from build123d import *

# Parameters (mm, degrees)
SKETCH2_R           = 6
BOSS_EXTRUDE1_DEPTH = 10
SKETCH3_W           = 75
SKETCH3_H           = 10
BOSS_EXTRUDE2_DEPTH = 60
SKETCH4_R           = 2.25
CUT_EXTRUDE1_DEPTH  = 9
SKETCH5_W           = 10
SKETCH5_H           = 10
CUT_EXTRUDE2_DEPTH  = 2.5


with BuildPart() as part:
    # Sketch2 → Boss-Extrude1 (new body)
    with BuildSketch(Plane.XY):
        with BuildLine():
            Line((-37.5, -5), (37.5, -5))
            Line((37.5, -5), (37.5, 5))
            Line((37.5, 5), (5.548671219, 35.763006828))
            ThreePointArc((5.548671219, 35.763006828), (0, 38), (-5.548671219, 35.763006828))
            Line((-5.548671219, 35.763006828), (-37.5, 5))
            Line((-37.5, 5), (-37.5, -5))
        make_face()
        with Locations((0, 30)):
            Circle(SKETCH2_R, mode=Mode.SUBTRACT)
    extrude(amount=BOSS_EXTRUDE1_DEPTH)

    # Sketch3 → Boss-Extrude2 (add)
    with BuildSketch(Plane.XY):
        Rectangle(SKETCH3_W, SKETCH3_H)
    extrude(amount=BOSS_EXTRUDE2_DEPTH)

    # Sketch4 → Cut-Extrude1 (cut)
    with BuildSketch(Plane.XZ.offset(5)):
        with Locations((27.5, 5)):
            Circle(SKETCH4_R)
        with Locations((12.5, 5)):
            Circle(SKETCH4_R)
        with Locations((-12.5, 5)):
            Circle(SKETCH4_R)
        with Locations((-27.5, 5)):
            Circle(SKETCH4_R)
    extrude(amount=-CUT_EXTRUDE1_DEPTH, mode=Mode.SUBTRACT)

    # Sketch5 → Cut-Extrude2 (cut)
    with BuildSketch(Plane(origin=(0, 0, 0), x_dir=(-1, 0, 0), z_dir=(0, 0, -1))):
        with Locations((-10, 5)):
            Rectangle(SKETCH5_W, SKETCH5_H)
        with Locations((10, 5)):
            Rectangle(SKETCH5_W, SKETCH5_H)
    extrude(amount=-CUT_EXTRUDE2_DEPTH, mode=Mode.SUBTRACT)


solid = part.part
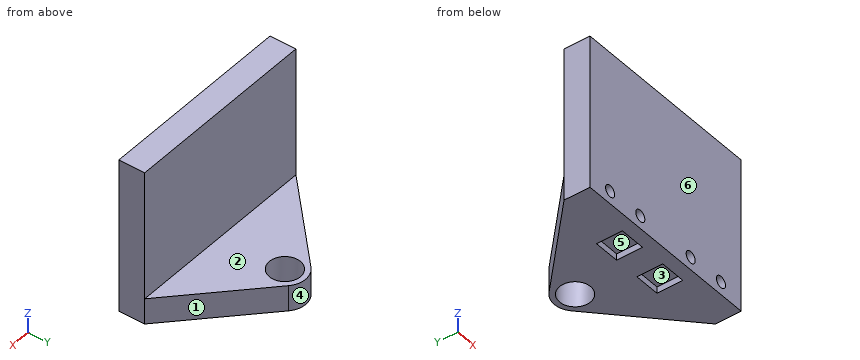
Here's how the part is built. I have some questions about the finished solid (model axes, mm). Face numbers are marked on the shaded views. A direction names the side the tool comes from. Give positions to 0.01 mm unless a question says otherwise; leave off trailing zeros. Loops run counter-clockwise (first coordinate to the right, second up) from the corner with the lowest first, then second, coordinate; pieces in that order, holes last. Notation, with made-up numbers: (57.25, -30.75) -> (85.25, -30.75) arc R31 ccw to (85.25, 7.25) -> close; hole circle Ø10 at (72, 40). An arc over 180 degrees is marked (long way). Answer as a JSON object with one key per item and string values. Group by question number.
Item 1: On a 3-axis mill with a long thin cutter (end or side, diameter ignored), from which of +Z, -Z, +X, -X, +Y, -Y can I reach the whole of each face in a straight line? I mean the marked faces 1, 2 and 3. Say none if no direction works.
Item 2: Imagine slicing it at D-D on x = 27.5. Write out the boundary of the cut face in (y, z).
Item 3: Thinking about a two-plate mould opening in X: for the marked faces 4, 5 and 6, which applies, pulls with the +X half, pulls with the -X half, needs draft (parallel to the pull), parting line crosses it, or undercut?
Item 4: Imagine slicing it at B-B on z = 5. Write out the boundary of the cut face in (x, y), then the cut area to 3 significant figures.
Item 5: Imagine slicing it at C-C on y = 27. Write out the boundary of the cut face in (x, z).
Item 6: Imagine slicing it at A-A on x = 0. Write out the boundary of the cut face in (y, z), then the cut area to 3 significant figures.
Item 7: Will these pins go through, and if not, where does the flat tip stop? pin 1 (2.5 mm diameter, centred on x = 27.5, z = 5, fed in from -Y); pin 2 (4 mm diameter, centred on x = -27.5, z = 5, fed in from +Y); pin 3 (1.5 mm diameter, centred on x = 12.5, y = 25.5, fed in from +Z); pin 4 (9.5 mm diameter, centred on x = 0, y = 30, fed in from -Z).
Item 8: I need wall thicknesses on L1, parallel to Z at x = -12.5, y = -0.75; L2, parallel to Z at x = -12.5, y = 1; L3, parallel to Y at x = -9.5, z = 53.5. Which ranges of each line are inside material? Lowest first, please.
Answer list:
{
 "1": {"face 1": "+Z, -Z, +X, +Y", "face 2": "+Z, +X, -X, +Y", "face 3": "-Z"},
 "2": {"outline": "(-5, 0) -> (14.63, 0) -> (14.63, 10) -> (5, 10) -> (5, 60) -> (-5, 60) -> (-5, 7.25) -> (4, 7.25) -> (4, 2.75) -> (-5, 2.75) -> close"},
 "3": {"face 4": "parting line crosses it", "face 5": "undercut", "face 6": "needs draft"},
 "4": {"outline": "(-37.5, -5) -> (-29.75, -5) -> (-29.75, 4) -> (-25.25, 4) -> (-25.25, -5) -> (-14.75, -5) -> (-14.75, 4) -> (-10.25, 4) -> (-10.25, -5) -> (10.25, -5) -> (10.25, 4) -> (14.75, 4) -> (14.75, -5) -> (25.25, -5) -> (25.25, 4) -> (29.75, 4) -> (29.75, -5) -> (37.5, -5) -> (37.5, 5) -> (5.55, 35.76) arc R8 ccw to (-5.55, 35.76) -> (-37.5, 5) -> close; hole circle Ø12 at (0, 30)", "area": "1,820 mm2"},
 "5": {"outline": "(-14.65, 0) -> (-5.2, 0) -> (-5.2, 10) -> (-14.65, 10) -> close; (5.2, 0) -> (14.65, 0) -> (14.65, 10) -> (5.2, 10) -> close"},
 "6": {"outline": "(-5, 0) -> (24, 0) -> (24, 10) -> (5, 10) -> (5, 60) -> (-5, 60) -> close; (36, 0) -> (38, 0) -> (38, 10) -> (36, 10) -> close", "area": "810 mm2"},
 "7": {"pin 1": "stops at y = 4", "pin 2": "stops at y = 16.55", "pin 3": "stops at z = 10", "pin 4": "passes through"},
 "8": {"L1": "z = 0 to 2.75, 7.25 to 60", "L2": "z = 2.5 to 2.75, 7.25 to 60", "L3": "y = -5 to 5"}
}
